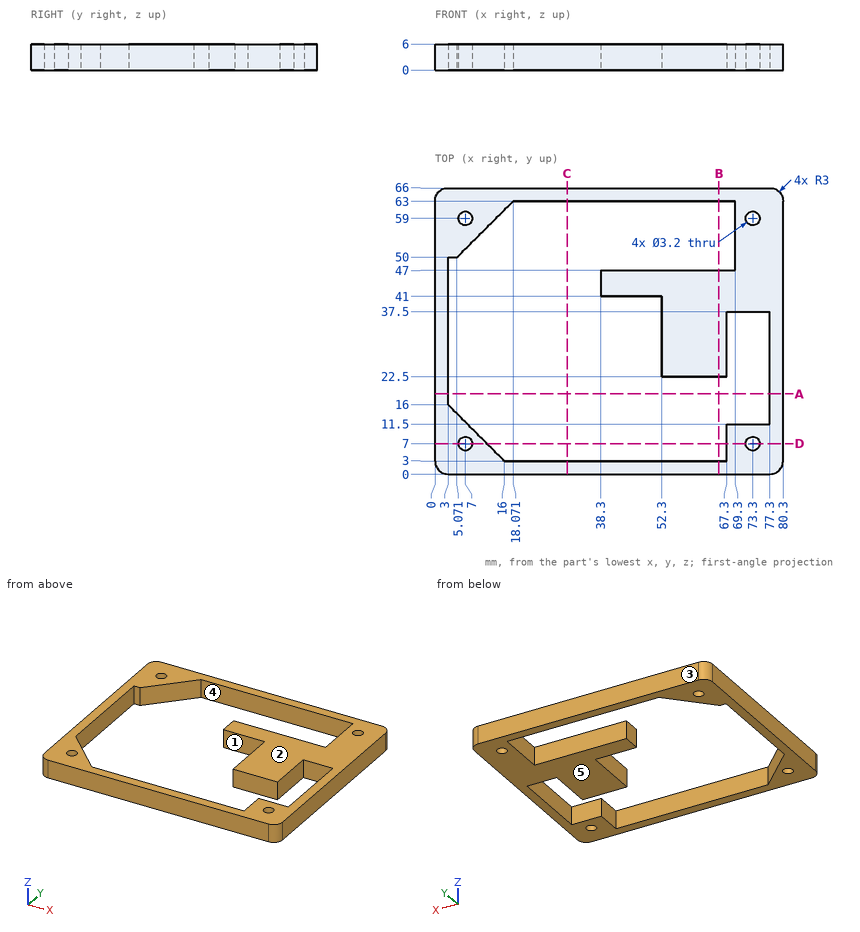
The drawing under review shows one solid part. Ordinate dimensions are in mm from its lowest x, y, z. A direction names the side the tool comes from. Coordinates: 2 decimals unless noted, no trailing zeros. Loops run counter-clockwise (first coordinate to the right, second up) from the corner with the lowest first, then second, coordinate; pieces in that order, holes last. Notation, with made-up numbers: (20, 35.5) - (34, 35.5) arc R18 cw to (34, 54.5) - close; hole circle Ø3 at (12, 64). An arc over 180 degrees is marked (long way). Use CSV: the item, a comma, the result in double quotes. Start each with the question number.
1. To check wall thickness, follow probe 1 along Y at (x, z) = (73.3, 4.5); probe 2 along Y at (x, z) = (64, 0.5); probe 3 along X at (y, z) = (26.5, 5.5). State the ranges of each line that lie inside material, in increasing order.
2. Mouldability with a two-part tool opening along Y and no side actions: class the marked faces 3, 4 and 5 as released by +Y, released by -Y, zero draft, split by the parting line, or undercut.
3. Add section B-B on x = 65.5. Give the boundary of the cut face in (y, z), plus the area to 3 significant figures.
4. Add section C-C on x = 30.5. Give the boundary of the cut face in (y, z).
5. Add section D-D on y = 7. Give the boundary of the cut face in (x, z).
6. For the marked faces 1 and 2, list the 3-axis set-ups (+Z, -Z, +X, -X, +Y, -Y) from which the entire face can be reached by the end or side of a thin tool; tool diameter is ignored.
7. Add section A-A on y = 18.5. Give the boundary of the cut face in (x, z), plus the area to 3 significant figures.
8. Clearance check with a flat-ended pin moving along its axis: pin 1 (3 mm diameter, centred on y = 22.5, z = 2.5, fed in from -X). State where the tip first meets the part, or that it passes through.
Resolved:
1,probe 1,"0 to 5.4, 8.6 to 11.5, 37.5 to 57.4, 60.6 to 66"
1,probe 2,"0 to 3, 22.5 to 47, 63 to 66"
1,probe 3,"0 to 3, 52.3 to 67.3, 77.3 to 80.3"
2,face 3,"released by +Y"
2,face 4,"undercut"
2,face 5,"zero draft"
3,outline,"(0, 0) - (3, 0) - (3, 6) - (0, 6) - close; (22.5, 0) - (47, 0) - (47, 6) - (22.5, 6) - close; (63, 0) - (66, 0) - (66, 6) - (63, 6) - close"
3,area,"183 mm2"
4,outline,"(0, 0) - (3, 0) - (3, 6) - (0, 6) - close; (63, 0) - (66, 0) - (66, 6) - (63, 6) - close"
5,outline,"(0, 0) - (5.4, 0) - (5.4, 6) - (0, 6) - close; (8.6, 0) - (12, 0) - (12, 6) - (8.6, 6) - close; (67.3, 0) - (71.7, 0) - (71.7, 6) - (67.3, 6) - close; (74.9, 0) - (80.3, 0) - (80.3, 6) - (74.9, 6) - close"
6,face 1,"+Z, -Z"
6,face 2,"+Z, +X, -X, +Y, -Y"
7,outline,"(0, 0) - (3, 0) - (3, 6) - (0, 6) - close; (77.3, 0) - (80.3, 0) - (80.3, 6) - (77.3, 6) - close"
7,area,"36.0 mm2"
8,pin 1,"x = 0"
